```python
from build123d import *

# Parameters (mm, degrees)
F0_W     = 19.275
F0_H     = 74.8
F0_R     = 1.75
F0_R_2   = 1.2
F1_DEPTH = 6
F3_DEPTH = 25
F2_R     = 1.2
F4_DEPTH = 3
F5_SIZE  = 3
F2_R_2   = 1.75
F6_DEPTH = 4
F7_R     = 3.5
F7_R_2   = 1.2
F8_DEPTH = 3


# Not quite as in the source:
# - a feature names something its author has since deleted; it is built from what else it names


with BuildPart() as f1:
    # F0 (on Top) → F1 (new body)
    with BuildSketch(Plane.XY):
        with Locations((-45.9428956378, 11.8681262247)):
            Rectangle(F0_W, F0_H)
        with Locations((-50.5803956378, -20.5318737753)):
            Circle(F0_R, mode=Mode.SUBTRACT)
        with Locations((-40.3053956378, -10.3568737753)):
            Circle(F0_R_2, mode=Mode.SUBTRACT)
        with Locations((-40.3053956378, 34.0931262247)):
            Circle(F0_R_2, mode=Mode.SUBTRACT)
        with Locations((-50.5803956378, 44.2681262247)):
            Circle(F0_R, mode=Mode.SUBTRACT)
    extrude(amount=F1_DEPTH)

    # F2 (on face) → F3 (cut)
    with BuildSketch(Plane.XY.offset(6)):
        Polygon((-47.307246298, 49.2681262247), (-41.8063209679, 43.7672008947), (-36.3053956378, 38.2662755646), (-36.3053956378, 49.2681262247), align=None)
        Polygon((-55.5803956378, 40.9949768848), (-55.5803956378, -17.2587244354), (-50.0794703078, -11.7577991053), (-46.5803956378, -8.2587244354), (-46.5803956378, 31.9949768848), (-50.0794703078, 35.4940515548), align=None)
        Polygon((-36.3053956378, -14.5300231152), (-41.8063209679, -20.0309484452), (-47.307246298, -25.5318737753), (-36.3053956378, -25.5318737753), align=None)
    extrude(amount=-F3_DEPTH, mode=Mode.SUBTRACT)

    # F2 (on face) → F4 (cut)
    with BuildSketch(Plane.XY.offset(6)):
        Polygon((-46.5803956378, -8.2587244354), (-50.0794703078, -11.7577991053), (-41.8063209679, -20.0309484452), (-36.3053956378, -14.5300231152), (-36.3053956378, 38.2662755646), (-41.8063209679, 43.7672008947), (-50.0794703078, 35.4940515548), (-46.5803956378, 31.9949768848), align=None)
        with Locations((-40.3053956378, -10.3568737753)):
            Circle(F2_R, mode=Mode.SUBTRACT)
        with Locations((-40.3053956378, 34.0931262247)):
            Circle(F2_R, mode=Mode.SUBTRACT)
    extrude(amount=-F4_DEPTH, mode=Mode.SUBTRACT)

    # F5
    f5_edges = [f1.edges().sort_by_distance(p)[0] for p in [
        (-55.580396, 49.268126, 3),
        (-55.580396, -25.531874, 3),
    ]]
    chamfer(f5_edges, length=F5_SIZE)

    # F2 (on face) → F6 (cut)
    with BuildSketch(Plane.XY.offset(6)):
        Polygon((-49.7286489393, 47.4468881789), (-52.9074108935, 46.5951414804), (-53.759157592, 43.4163795262), (-51.4321423364, 41.0893642705), (-48.2533803822, 41.9411109691), (-47.4016336836, 45.1198729233), align=None)
        with Locations((-50.5803956378, 44.2681262247)):
            Circle(F2_R_2, mode=Mode.SUBTRACT)
        Polygon((-52.9074108935, -22.8588890309), (-49.7286489393, -23.7106357295), (-47.4016336836, -21.3836204738), (-48.2533803822, -18.2048585196), (-51.4321423364, -17.3531118211), (-53.759157592, -19.6801270767), align=None)
        with Locations((-50.5803956378, -20.5318737753)):
            Circle(F2_R_2, mode=Mode.SUBTRACT)
    extrude(amount=-F6_DEPTH, mode=Mode.SUBTRACT)

    # F7 (on face) → F8 (join)
    with BuildSketch(Plane.XY.offset(3)):
        with Locations((-40.3053956378, -10.3568737753)):
            Circle(F7_R)
        with Locations((-40.3053956378, -10.3568737753)):
            Circle(F7_R_2, mode=Mode.SUBTRACT)
        with Locations((-40.3053956378, 34.0931262247)):
            Circle(F7_R)
        with Locations((-40.3053956378, 34.0931262247)):
            Circle(F7_R_2, mode=Mode.SUBTRACT)
    extrude(amount=F8_DEPTH)


solid = f1.part
```
Work out the finished part from the listing and answer in its coordinate system (mm). A direction names the side the tool comes from. Give positions to 0.01 mm unless a question says otherwise; leave off trailing zeros. Loops run counter-clockwise (first coordinate to the right, second up) from the corner with the lowest first, then second, coordinate; pieces in that order, holes last. Notation, with made-up numbers: (50, 60.25) -> (93, 60.25) arc R32 ccw to (93, 86.25) -> close; hole circle Ø10 at (15.5, 38). An arc over 180 degrees is marked (long way). Put each result on its own line as item: value. Start each with the question number.
Item 1: Which of the six approach directions +Z, -Z, +X, -X, +Y, -Y give full straight-line access (tool end or side, diameter ignored) to faces 5 (the face through (-42.885, 36.459, 4.479)), 6 (the face through (-46.58, 12, 2)), 7 (the face through (-36.305, 11, 1))?
Item 2: The part is cut by section B-B (y = -4). Give the vertices of the cut face in (x, z), then the cut area to 3 significant figures.
Item 3: Each of these flat-tipped pins is pushed along its axis until it touches: P1, Ø3, axis at x = -51.5, y = -20.5, coming from the +Z side; P2, Ø2, axis at x = -40.31, y = 34.09, coming from the -Z side; P3, Ø5, axis at x = -44.5, y = 18.5, coming from the +Z side; P4, Ø3.5, axis at y = 19, z = 1.5, coming from the -X side. Where does it stop, or does it pass through?
Item 4: The mould has two halves that part along X. Classify faces 1 (the face through (-43.8, -10.2, 4.5)), 2 (the face through (-54.06, 47.79, 2.96)), 3 (the face through (-50, -17, 6)), 4 (the face through (-48.91, -20.01, 0.99)): released by +X, released by -X, zero draft, split by the parting line, or undercut.
Item 5: The part is cut by section A-A (z = 1). Give the vertices of the cut face in (x, y), then the cut area to 3 significant figures.
Item 6: Find the intervals of material crossed by L1, parallel to Y at x = -40, z = 1.5; L2, parallel to Y at x = -42.75, z = 4.75; L3, parallel to Y at x = -51.25, z = 5, in increasing order. Write a range as [from, to].
Item 7: The part is cut by section C-C (x = -38.25). Give the vertices of the cut face in (y, z).
Answers below:
1. face 5: +Z
1. face 6: +Z, -Z, -X
1. face 7: +Z, -Z, +X, +Y, -Y
2. outline: (-46.58, 0) -> (-36.31, 0) -> (-36.31, 3) -> (-46.58, 3) -> close
2. area: 30.8 mm2
3. P1: z = 2
3. P2: through
3. P3: z = 3
3. P4: x = -46.58
4. face 1: undercut
4. face 2: released by -X
4. face 3: zero draft
4. face 4: undercut
5. outline: (-55.58, -22.53) -> (-52.58, -25.53) -> (-47.31, -25.53) -> (-36.31, -14.53) -> (-36.31, 38.27) -> (-47.31, 49.27) -> (-52.58, 49.27) -> (-55.58, 46.27) -> (-55.58, 40.99) -> (-46.58, 31.99) -> (-46.58, -8.26) -> (-55.58, -17.26) -> close; hole circle Ø3.5 at (-50.58, -20.53); hole circle Ø3.5 at (-50.58, 44.27); hole circle Ø2.4 at (-40.31, -10.36); hole circle Ø2.4 at (-40.31, 34.09)
5. area: 840 mm2
6. L1: [-18.22, -11.52], [-9.2, 32.93], [35.25, 41.96]
6. L2: [-20.97, -19.09], [-12.86, -7.85], [31.59, 36.6], [42.82, 44.71]
6. L3: [-25.53, -23.3], [-17.4, -12.93], [36.66, 41.14], [47.04, 49.27]
7. outline: (-16.47, 0) -> (40.21, 0) -> (40.21, 3) -> (36.93, 3) -> (36.93, 6) -> (31.26, 6) -> (31.26, 3) -> (-7.52, 3) -> (-7.52, 6) -> (-13.19, 6) -> (-13.19, 3) -> (-16.47, 3) -> close
